from build123d import *

# Parameters (mm, degrees)
SKETCH2_R           = 20
BOSS_EXTRUDE2_DEPTH = 5
SKETCH3_W           = 5
SKETCH3_H           = 5
BOSS_EXTRUDE3_DEPTH = 43
SKETCH4_R           = 2.5
BOSS_EXTRUDE4_DEPTH = 41
SKETCH5_W           = 7.704684196
SKETCH5_H           = 10
CUT_EXTRUDE1_DEPTH  = 52.46843693
FILLET1_R           = 2
CHAMFER1_SIZE       = 1
SKETCH6_W           = 43
SKETCH6_H           = 5
CUT_EXTRUDE2_DEPTH  = 0.2
SKETCH7_W           = 43
SKETCH7_H           = 5
CUT_EXTRUDE3_DEPTH  = 0.2


with BuildPart() as part:
    # Sketch2 → Boss-Extrude2 (new body)
    with BuildSketch(Plane(origin=(0, 0, 0), x_dir=(0, 0, -1), z_dir=(1, 0, 0))):
        Circle(SKETCH2_R)
    extrude(amount=BOSS_EXTRUDE2_DEPTH)

    # Sketch3 → Boss-Extrude3 (add)
    with BuildSketch(Plane(origin=(5, 0, 0), x_dir=(0, 0, -1), z_dir=(1, 0, 0))):
        Rectangle(SKETCH3_W, SKETCH3_H)
    extrude(amount=BOSS_EXTRUDE3_DEPTH)

    # Sketch4 → Boss-Extrude4 (add)
    with BuildSketch(Plane(origin=(5, 0, 0), x_dir=(0, 0, -1), z_dir=(1, 0, 0))):
        with Locations((-8.485281374, 8.485281374)):
            Circle(SKETCH4_R)
        with Locations((8.485281374, -8.485281374)):
            Circle(SKETCH4_R)
    extrude(amount=BOSS_EXTRUDE4_DEPTH)

    # Sketch5 → Cut-Extrude1 (cut, through all)
    with BuildSketch(Plane(origin=(5, 0, 0), x_dir=(0, 0, -1), z_dir=(1, 0, 0))):
        with BuildLine():
            Line((-12, 16), (-3.852342098, 16))
            Line((-3.852342098, 16), (-3.852342098, 19.625479876))
            ThreePointArc((-3.852342098, 19.625479876), (-8.130818752, 18.272651324), (-12, 16))
        make_face()
        with BuildLine():
            Line((-3.852342098, 19.625479876), (-3.852342098, 16))
            Line((-3.852342098, 16), (3.852342098, 16))
            Line((3.852342098, 16), (3.852342098, 19.625479876))
            ThreePointArc((3.852342098, 19.625479876), (1.935252254, 19.906149771), (2.3e-08, 20))
            ThreePointArc((2.3e-08, 20), (-1.935252231, 19.906149773), (-3.852342098, 19.625479876))
        make_face()
        with BuildLine():
            Line((3.852342098, 19.625479876), (3.852342098, 16))
            Line((3.852342098, 16), (12, 16))
            ThreePointArc((12, 16), (8.130818752, 18.272651324), (3.852342098, 19.625479876))
        make_face()
        with Locations((0, 11)):
            Rectangle(SKETCH5_W, SKETCH5_H)
    extrude(amount=-CUT_EXTRUDE1_DEPTH, mode=Mode.SUBTRACT)

    # Fillet1
    fillet1_edges = [part.edges().sort_by_distance(p)[0] for p in [
        (2.5, 16, 12),
        (2.5, 16, -12),
        (2.5, 16, -3.852342098),
        (2.5, 16, 3.852342098),
    ]]
    fillet(fillet1_edges, radius=FILLET1_R)

    # Chamfer1
    chamfer1_edges = [part.edges().sort_by_distance(p)[0] for p in [
        (5, 8.485281374, 10.985281374),
        (5, -8.485281374, -5.985281374),
    ]]
    chamfer(chamfer1_edges, length=CHAMFER1_SIZE)

    # Sketch6 → Cut-Extrude2 (cut)
    with BuildSketch(Plane(origin=(0, 0, -2.5), x_dir=(-1, 0, 0), z_dir=(0, 0, -1))):
        with Locations((-26.5, 0)):
            Rectangle(SKETCH6_W, SKETCH6_H)
    extrude(amount=-CUT_EXTRUDE2_DEPTH, mode=Mode.SUBTRACT)

    # Sketch7 → Cut-Extrude3 (cut)
    with BuildSketch(Plane.XY.offset(2.5)):
        with Locations((26.5, 0)):
            Rectangle(SKETCH7_W, SKETCH7_H)
    extrude(amount=-CUT_EXTRUDE3_DEPTH, mode=Mode.SUBTRACT)


solid = part.part
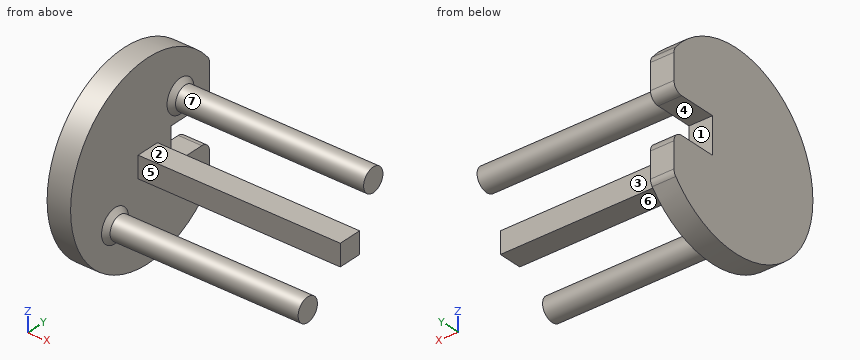
Could you check a few things on this model? Use its own coordinates, in mm. Face numbers are marked on the shaded views. A direction names the side the tool comes from. Give positions to 0.01 mm unless a question says otherwise; leave off trailing zeros. Order: outer loops, then holes, each group sorted by start corner. A loop starts at its lowest first (then second) coordinate and runs counter-clockwise, first axis right, second up. Notation, with made-up numbers: (-27.75, -33.5) - (10.25, -33.5) arc R12 cw to (10.25, -19.5) - close; hole circle Ø3 at (49.5, -35). An arc over 180 degrees is marked (long way). Return JSON: item names as keys, results as strings. Group by question number.
Q1. Suppose I cut it at B-B, the plane z = 0. Please give me the cut outline in (x, y).
Q2. Will these pins go through, and if not, where does the flat tip stop? pin 1 Ø1.4 at (x, z) = (22.5, 0) entering from +Y; pin 2 Ø8 at (x, y) = (41.5, -1) entering from -Z; pin 3 Ø1.5 at (y, z) = (2.5, -11.5) entering from +X; pin 4 Ø18 at (y, z) = (-8, -5) entering from +X.
Q3. Suppose I cut it at D-D, the plane x = 44. Please give me the cut outline in (y, z), and give its area (3 significant figures).
Q4. Suppose I cut it at C-C, the plane y = 0. Please give me the cut outline in (x, z).
Q5. Please list where these lines run through material, in increasing order: line 1 along X through (y, z) = (11.5, 15); line 2 along Y through (x, z) = (10, 0); line 3 along Z through (x, y) = (40.5, 1). Write a range as [from, to].
Q6. Suppose I cut it at A-A, the plane x = 4. Please give me the cut outline in (y, z), and give its area (3 significant figures).
Q7. Which directions (+Z, -Z, +X, -X, +Y, -Y) give clear straight access to the entire face, cutting with the end or side of a thin tool? Please do the marked faces 5, 6 and 7.
Q8. Thinking about a two-plate mould opening in Z: for the marked faces 1, 2, 3 and 4, which applies, pulls with the +Z half, pulls with the -Z half, needs draft (parallel to the pull), parting line crosses it, or undercut?
Resolved:
{
 "1": {"outline": "(0, -20) - (5, -20) - (5, -2.5) - (48, -2.5) - (48, 2.5) - (5, 2.5) - (5, 6) - (0, 6) - close"},
 "2": {"pin 1": "stops at y = 2.5", "pin 2": "stops at z = -2.3", "pin 3": "stops at x = 5", "pin 4": "stops at x = 48"},
 "3": {"outline": "circle Ø5 at (-8.49, -8.49); (-2.5, -2.3) - (2.5, -2.3) - (2.5, 2.3) - (-2.5, 2.3) - close; circle Ø5 at (8.49, 8.49)", "area": "62.3 mm2"},
 "4": {"outline": "(0, -20) - (5, -20) - (5, -2.3) - (48, -2.3) - (48, 2.3) - (5, 2.3) - (5, 20) - (0, 20) - close"},
 "5": {"line 1": "x = [0, 5]", "line 2": "y = [-2.5, 2.5]", "line 3": "z = [-2.3, 2.3]"},
 "6": {"outline": "(6, -3.85) - (6, 3.85) - (14, 3.85) arc R2 ccw to (16, 5.85) - (16, 11.31) arc R2 ccw to (15.56, 12.57) arc R20 ccw (long way) to (15.56, -12.57) arc R2 ccw to (16, -11.31) - (16, -5.85) arc R2 ccw to (14, -3.85) - close", "area": "1,110 mm2"},
 "7": {"face 5": "+Z, -Z, +X, -Y", "face 6": "-Z, +X, +Y, -Y", "face 7": "+X"},
 "8": {"face 1": "undercut", "face 2": "pulls with the +Z half", "face 3": "needs draft", "face 4": "undercut"}
}
